from build123d import *

# Parameters (mm, degrees)
EXTRUDE1_DEPTH          = 12.7
F_1_4_CLEARANCE_HOLE1_D = 6.7564
F_1_4_CLEARANCE_HOLE2_D = 6.7564
FILLET1_R               = 2.54


with BuildPart() as part:
    # Sketch1 → Extrude1 (new, symmetric)
    with BuildSketch(Plane(origin=(0, 0, 0), x_dir=(0, 0, -1), z_dir=(1, 0, 0))):
        Polygon((0, 0), (0, 25.4), (3.175, 25.4), (3.175, 3.175), (25.4, 3.175), (25.4, 0), align=None)
    extrude(amount=EXTRUDE1_DEPTH, both=True)

    # 1/4 Clearance Hole1 (through all)
    with Locations(Plane.XY):
        with Locations((0, 12.7)):
            Hole(F_1_4_CLEARANCE_HOLE1_D / 2)

    # 1/4 Clearance Hole2 (through all)
    with Locations(Plane.XZ):
        with Locations((0, -12.7)):
            Hole(F_1_4_CLEARANCE_HOLE2_D / 2)

    # Fillet1
    fillet1_edges = [part.edges().sort_by_distance(p)[0] for p in [
        (0, 25.4, -3.175),
        (0, 3.175, -3.175),
        (0, 3.175, -25.4),
    ]]
    fillet(fillet1_edges, radius=FILLET1_R)


solid = part.part
Work out the finished part from the listing and answer in its coordinate system (mm). A direction names the side the tool comes from. Give positions to 0.01 mm unless a question says otherwise; leave off trailing zeros. Write each loop counter-clockwise with the first axis right and the second up, starting at its lowest first coordinate (ties: lowest second). Pieces come first, ordered by that corner, then holes. Notation, with made-up numbers: (54, 83) - (90, 83) arc R23 ccw to (90, 106) - close; hole circle Ø1 at (-28.5, 59). An arc over 180 degrees is marked (long way). One line per item, written item: value. Start each with the question number.
1. Find section D-D (x = -7.5). Write down the section's boundary in (y, z) (3 decimals), then the cut area to 3 significant figures.
2. Find section C-C (z = -12.7). Write down the section's boundary in (x, y) (3 decimals), then the cut area to 3 significant figures.
3. Given pin 1 (11 mm diameter, centred on x = 0, z = -12.7, fed in from +Y) (3 decimals); pin 2 (8.5 mm diameter, centred on x = 2.5, y = 13, fed in from -Z) (3 decimals), each flat-ended and moving along its own axis, determine where each tip first touches the part or whether it passes through.
4. For faces 1 (the flat face through (3, 3.175, -16)), 2 (the flat face through (-12.7, 2, -7)), determine the directions among +Z, -Z, +X, -X, +Y, -Y from which every point of the face is accessible in a straight line to the end or side of a thin tool.
5. For a pull along Y with two mould halves and no side action, classify faces 3 (the cylindrical face through (0.73, 9.4, -1.61)), 4 (the flat face through (0.2, 16.3, -3.175)), 5 (the cylindrical face through (0, 2, -25)) as +Y half, -Y half, draft (parallel to the pull), parting line (faces both ways), or undercut.
6. Consider probe 1 along Z at (x, y) = (9.5, 18.75) (3 decimals); probe 2 along Y at (x, z) = (-6.75, -14.75) (3 decimals); probe 3 along Y at (x, z) = (0, -1.7). Determine where each line is inside the solid, lowest interval first.
7. Find section A-A (x = 0). Write down the section's boundary in (y, z) (3 decimals).
8. Find section B-B (y = 12.7). Write down the section's boundary in (x, z) (3 decimals), then the cut area to 3 significant figures.
Geometry results:
1. outline: (0, -25.4) - (0.635, -25.4) arc R2.54 ccw to (3.175, -22.86) - (3.175, -5.715) arc R2.54 cw to (5.715, -3.175) - (22.86, -3.175) arc R2.54 ccw to (25.4, -0.635) - (25.4, 0) - (0, 0) - close
1. area: 150 mm2
2. outline: (-12.7, 0) - (-3.378, 0) - (-3.378, 3.175) - (-12.7, 3.175) - close; (3.378, 0) - (12.7, 0) - (12.7, 3.175) - (3.378, 3.175) - close
2. area: 59.2 mm2
3. pin 1: y = 3.175
3. pin 2: z = -3.175
4. face 1: -Z, +X, -X, +Y
4. face 2: +Z, -Z, -X, +Y, -Y
5. face 3: undercut
5. face 4: draft
5. face 5: +Y half
6. probe 1: -3.175 to 0
6. probe 2: 0 to 3.175
6. probe 3: 0 to 9.32, 16.08 to 25.17
7. outline: (0, -25.4) - (0.635, -25.4) arc R2.54 ccw to (3.175, -22.86) - (3.175, -16.078) - (0, -16.078) - close; (0, -9.322) - (3.175, -9.322) - (3.175, -5.715) arc R2.54 cw to (5.715, -3.175) - (9.322, -3.175) - (9.322, 0) - (0, 0) - close; (16.078, -3.175) - (22.86, -3.175) arc R2.54 ccw to (25.4, -0.635) - (25.4, 0) - (16.078, 0) - close
8. outline: (-12.7, -3.175) - (-3.378, -3.175) - (-3.378, 0) - (-12.7, 0) - close; (3.378, -3.175) - (12.7, -3.175) - (12.7, 0) - (3.378, 0) - close
8. area: 59.2 mm2
